from build123d import *

# Parameters (mm, degrees)
F0_W        = 127
F0_H        = 76.2
F0_R        = 7.0531122836
F0_R_2      = 6.35
F1_DEPTH    = 50.8
F2_R        = 10.5798439837
F3_DEPTH    = 86.868
F4_T1_DEPTH = 192.3207478943
F5_R        = 12.7


# Not quite as in the source:
# - a fillet or chamfer that OpenCascade refuses, or shapes differently, is made with other operations: its cross-section is extruded or revolved along the edge and cut away or added


with BuildPart() as f1:
    # F0 (on Front) → F1 (new body)
    with BuildSketch(Plane.XZ):
        with Locations((0.679500401, -0.9445134997)):
            Rectangle(F0_W, F0_H)
        with Locations((-49.6532134712, 14.4240399823)):
            Circle(F0_R, mode=Mode.SUBTRACT)
        with Locations((45.129500401, 11.7554865003)):
            Circle(F0_R_2, mode=Mode.SUBTRACT)
    extrude(amount=F1_DEPTH)

    # F2 (on face) → F3 (cut)
    with BuildSketch(Plane.XZ.offset(50.8)):
        with Locations((-27.3451898247, 14.4321834669)):
            Circle(F2_R)
    extrude(amount=-F3_DEPTH, mode=Mode.SUBTRACT)

    # F4: chamfer of 12.7 on 1 edges, made by hand

    # F4_s2 → F4_t1 (cut)
    with BuildSketch(Plane.YZ.offset(-95.4808735461)):
        Polygon((-38.1, 37.1554865003), (-50.8, 24.4554865003), (-50.8, 37.1554865003), align=None)
    extrude(amount=F4_T1_DEPTH, mode=Mode.SUBTRACT)

    # F5
    f5_edges = [f1.edges().sort_by_distance(p)[0] for p in [
        (-62.8205, -19.05, 37.155487),
    ]]
    fillet(f5_edges, radius=F5_R)


solid = f1.part
Could you check a few things on this model? Use its own coordinates, in mm. Coordinates: 2 decimals unless noted, no trailing zeros. Order: outer loops, then holes, each group sorted by start corner. A loop starts at its lowest first (then second) coordinate and runs counter-clockwise, first axis right, second up. Notation, with made-up numbers: (81, 7.25) -> (132, 7.25) arc R19 cw to (132, 18.25) -> close; hole circle Ø11 at (-39, 30). An arc over 180 degrees is marked (long way). One line per item, written item: value. Start each with the question number.
1) Imagine slicing it at A-A on x = 19. List the corners of the cut face in (y, z) for me.
2) Imagine slicing it at B-B on y = -4. List the corners of the cut face in (x, z) for me.
3) If I drill on L1, parallel to X at y = -17.5, z = 19; L2, parallel to X at y = -38.5, z = 9.5; L3, parallel to X at y = -45, z = 7, over which ranges is the centre line in solid material (lowest first)? Write a range as [from, to].
4) Imagine slicing it at C-C on z = 28. List the corners of the cut face in (x, y) for me.
5) I'm going to push flat-ended pins straight in: pin 1 (3 mm diameter, centred on x = 23, z = 28.5, fed in from -Y); pin 2 (6 mm diameter, centred on x = -7, y = -42, fed in from +Z); pin 3 (8 mm diameter, centred on x = 27, y = -44.5, fed in from +Z); pin 4 (12.5 mm diameter, centred on x = -27.35, z = 14.43, fed in from +Y). Where does each tip first touch, or does it pass through?
6) We'd pull the mould along X, two halves only. Please class faces 1 (the flat face through (64.18, -25, -1)), 2 (the cylindrical face through (38.786, -25.044, 12.035)), 3 (the flat face through (0, -25, -39.045)): +X half, -X half, draft (parallel to the pull), parting line (faces both ways), or undercut.
Answer list:
1. outline: (-50.8, -39.04) -> (0, -39.04) -> (0, 37.16) -> (-38.1, 37.16) -> (-50.8, 24.46) -> close
2. outline: (-62.82, -39.04) -> (64.18, -39.04) -> (64.18, 37.16) -> (-50.12, 37.16) arc R12.7 ccw to (-62.82, 24.46) -> close; hole circle Ø14.11 at (-49.65, 14.42); hole circle Ø21.16 at (-27.35, 14.43); hole circle Ø12.7 at (45.13, 11.76)
3. L1: x = [-62.82, -55.02], [-44.29, -36.89], [-17.8, 64.18]
3. L2: x = [-62.82, -54.7], [-44.6, -36.71], [-17.99, 39.19], [51.07, 64.18]
3. L3: x = [-62.82, -34.87], [-19.82, 40.92], [49.34, 64.18]
4. outline: (-62.32, -47.26) -> (64.18, -47.26) -> (64.18, 0) -> (-62.32, 0) -> close
5. pin 1: stops at y = -48.26
5. pin 2: stops at z = 36.26
5. pin 3: stops at z = 34.76
5. pin 4: passes through
6. face 1: +X half
6. face 2: undercut
6. face 3: draft
